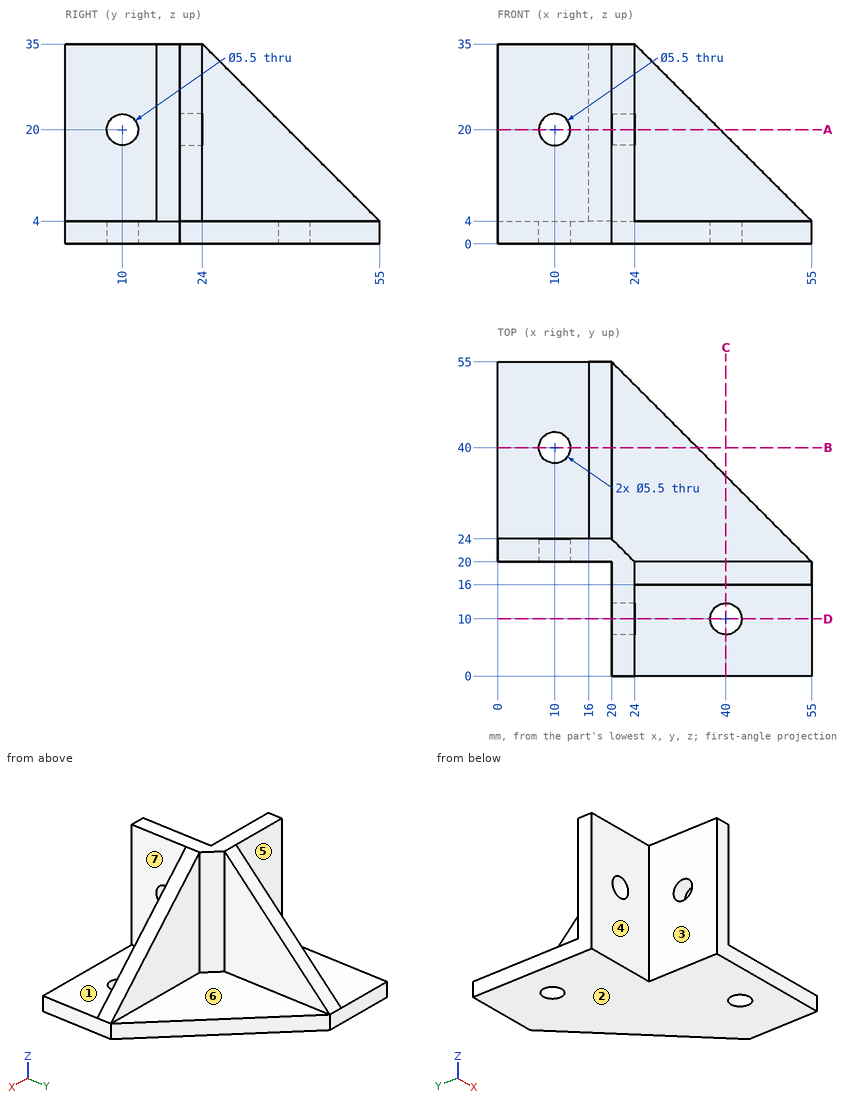
Geometry check sheet. Reference: drawing and pictorial views, mm from the part's lowest x, y, z. A direction names the side the tool comes from. Give positions to 0.01 mm unless a question says otherwise; leave off trailing zeros. Order: outer loops, then holes, each group sorted by start corner. A loop starts at its lowest first (then second) coordinate and runs counter-clockwise, first axis right, second up. Notation, with made-up numbers: M 77,41.25 L 104,41.25 A20 ccw 104,62.25 Z; hole C 4.25,51 d8. An arc over 180 degrees is marked long. Answer in a Markdown table with one row per item. Add a question column.
Item 1: Section check A-A, the plane z = 20. Enter the section's corners in (x, y), and give its area (3 significant figures).
Item 2: Gauge pin test, flat ends, axial feed: pin 1 (12 mm diameter, centred on x = 7, y = 49.5, fed in from +Z); pin 2 (1.5 mm diameter, centred on y = 7, z = 7, fed in from +X); pin 3 (4.5 mm diameter, centred on x = 10, z = 20, fed in from +Y); pin 4 (9.5 mm diameter, centred on x = 41.5, z = 17.5, fed in from +Y). Record the tip position at first contact, or that the pin passes through.
Item 3: Scan lines: probe 1 along Y at (x, z) = (40, 2.95); probe 2 along X at (y, z) = (36.5, 21); probe 3 along Y at (x, z) = (10, 1.8). Record each from-to range of solid material in increasing order. Write a range as from..to.
Item 4: Mould release check, pull along Z, two halves, no side actions. Record for the marked faces 1, 2 and 3: released by +Z, released by -Z, zero draft, split by the parting line, or undercut.
Item 5: Section check B-B, the plane y = 40. Enter the section's corners in (x, z), and give its area (3 significant figures).
Item 6: Tool access check on the marked faces 4, 5, 6 and 7. Record the directions out of +Z, -Z, +X, -X, +Y, -Y that give a thin tool (end or side, any length) a straight path to the whole face; none if there is none.
Item 7: Section check D-D, the plane y = 10. Enter the section's corners in (x, z), and give its area (3 significant figures).
Filled sheet:
| question | item | result |
|---|---|---|
| 1 | outline | M 0,20 L 7.25,20 L 7.25,24 L 0,24 Z; M 12.75,20 L 20,20 L 20,12.75 L 24,12.75 L 24,16 L 39,16 L 39,20 L 24,20 L 20,24 L 20,39 L 16,39 L 16,24 L 12.75,24 Z; M 20,0 L 24,0 L 24,7.25 L 20,7.25 Z |
| 1 | area | 244 mm^2 |
| 2 | pin 1 | stops at z = 4 |
| 2 | pin 2 | stops at x = 24 |
| 2 | pin 3 | passes through |
| 2 | pin 4 | stops at y = 20 |
| 3 | probe 1 | y = 0..7.25, 12.75..35 |
| 3 | probe 2 | x = 16..20 |
| 3 | probe 3 | y = 20..37.25, 42.75..55 |
| 4 | face 1 | released by +Z |
| 4 | face 2 | released by -Z |
| 4 | face 3 | zero draft |
| 5 | outline | M 0,0 L 7.25,0 L 7.25,4 L 0,4 Z; M 12.75,0 L 35,0 L 35,4 L 20,4 L 20,19 L 16,19 L 16,4 L 12.75,4 Z |
| 5 | area | 178 mm^2 |
| 6 | face 4 | +Z, -Z, -X, -Y |
| 6 | face 5 | +Z, -X, +Y |
| 6 | face 6 | +Z, +X, +Y |
| 6 | face 7 | +Z, +X, -Y |
| 7 | outline | M 20,0 L 37.25,0 L 37.25,4 L 24,4 L 24,17.25 L 20,17.25 Z; M 20,22.75 L 24,22.75 L 24,35 L 20,35 Z; M 42.75,0 L 55,0 L 55,4 L 42.75,4 Z |
| 7 | area | 220 mm^2 |
